```python
from build123d import *

# Parameters (mm, degrees)
PAD_DEPTH    = 9
POCKET_DEPTH = 6


with BuildPart() as part:
    # Sketch → Pad (new body)
    with BuildSketch(Plane.XY):
        with BuildLine():
            ThreePointArc((-89, 41), (-130, 0), (-89, -41))
            Line((-89, -41), (89, -41))
            ThreePointArc((89, -41), (130, 0), (89, 41))
            Line((-89, 41), (89, 41))
        make_face()
    extrude(amount=PAD_DEPTH)

    # Sketch001 (on Face6 of Pad) → Pocket (cut)
    with BuildSketch(Plane.XY.offset(9)):
        with BuildLine():
            ThreePointArc((-62.5, 6), (-68.5, 0), (-62.5, -6))
            Line((-62.5, -6), (62.5, -6))
            ThreePointArc((62.5, -6), (68.5, 0), (62.5, 6))
            Line((-62.5, 6), (62.5, 6))
        make_face()
    extrude(amount=-POCKET_DEPTH, mode=Mode.SUBTRACT)


solid = part.part
```
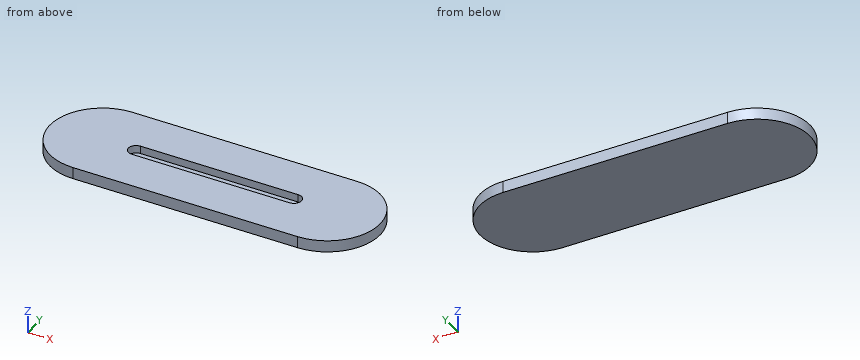
For this review, take the finished solid that the model builds, in its own axes (mm). Coordinates: 2 decimals unless noted, no trailing zeros. Loops run counter-clockwise (first coordinate to the right, second up) from the corner with the lowest first, then second, coordinate; pieces in that order, holes last.
1. Insertion check: P1, Ø1.5, axis at y = -24, z = 7.5, coming from the +X side; P2, Ø5, axis at x = 23, y = 5.5, coming from the -Z side; P3, Ø4, axis at y = -24, z = 5.5, coming from the +X side; P4, Ø1, axis at y = -9.5, z = 8, coming from the +X side. Each pin has a flat end and moves straight along its axis. Give the tip position at first contact, or say it passes through.
2. Add section C-C, the plane x = 111. Give the boundary of the cut face in (y, z).
3. Add section B-B, the plane y = 0. Give the boundary of the cut face in (x, z), then the cut area to 3 significant figures.
4. For line 1 (Y direction, x = -32.5, z = 4.75); line 2 (Y direction, x = -89.5, z = 2.75); line 3 (Z direction, x = -35.5, y = 1.5), list the stretches that pass through material, from the lowest coordinate up.
5. Add section D-D, the plane y = 32.5. Give the boundary of the cut face in (x, z) (3 decimals), then the cut area to 3 significant figures.
6. Add section A-A, the plane z = 6. Give the boundary of the cut face in (x, y).
Result:
1. P1: stops at x = 122.77
1. P2: stops at z = 0
1. P3: stops at x = 123.6
1. P4: stops at x = 129
2. outline: (-34.6, 0) - (34.6, 0) - (34.6, 9) - (-34.6, 9) - close
3. outline: (-130, 0) - (130, 0) - (130, 9) - (68.5, 9) - (68.5, 3) - (-68.5, 3) - (-68.5, 9) - (-130, 9) - close
3. area: 1,520 mm2
4. line 1: y = -41 to -6, 6 to 41
4. line 2: y = -41 to 41
4. line 3: z = 0 to 3
5. outline: (-113.995, 0) - (113.995, 0) - (113.995, 9) - (-113.995, 9) - close
5. area: 2,050 mm2
6. outline: (-89, -41) - (89, -41) arc R41 ccw to (89, 41) - (-89, 41) arc R41 ccw to start; hole (-62.5, -6) - (62.5, -6) arc R6 ccw to (62.5, 6) - (-62.5, 6) arc R6 ccw to start
